Could you check a few things on this drawing? It's one solid part, dimensions in mm from its lowest x, y, z. Give positions to 0.01 mm unless a question says otherwise; leave off trailing zeros. Order: outer loops, then holes, each group sorted by start corner. A loop starts at its lowest first (then second) coordinate and runs counter-clockwise, first axis right, second up. Notation, with made-up numbers: (2.25, -10) -> (9.25, -10) arc R16 cw to (9.25, 13) -> close; hole circle Ø1 at (-37, 19). An arc over 180 degrees is marked (long way). Answer as a JSON object with one key per item and string values.
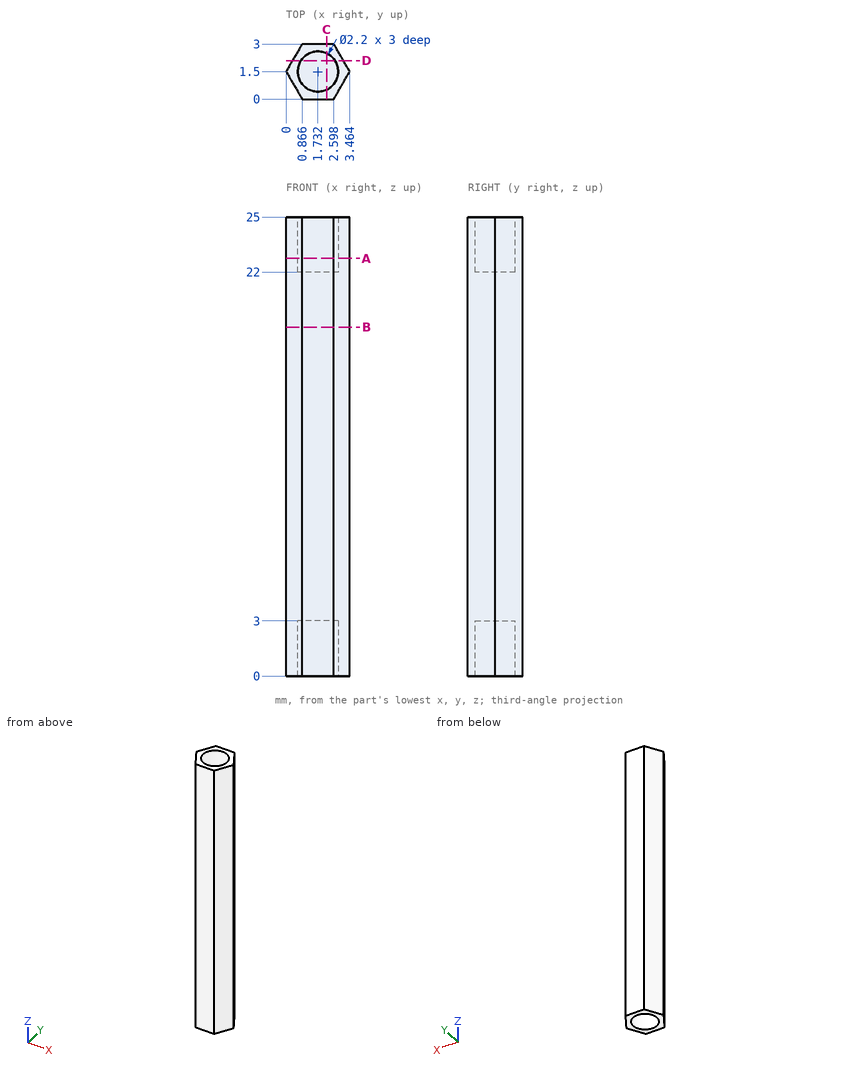
1. If we section it at A-A on z = 22.75: Please give me the cut outline in (x, y).
Worked answers:
{"outline": "(0, 1.5) -> (0.87, 0) -> (2.6, 0) -> (3.46, 1.5) -> (2.6, 3) -> (0.87, 3) -> close; hole circle Ø2.2 at (1.73, 1.5)"}
2. If we section it at B-B on z = 19: Please give me the cut outline in (x, y).
Worked answers:
{"outline": "(0, 1.5) -> (0.87, 0) -> (2.6, 0) -> (3.46, 1.5) -> (2.6, 3) -> (0.87, 3) -> close"}
3. If we section it at C-C on x = 2.2: Please give me the cut outline in (y, z).
Worked answers:
{"outline": "(0, 0) -> (0.5, 0) -> (0.5, 3) -> (2.5, 3) -> (2.5, 0) -> (3, 0) -> (3, 25) -> (2.5, 25) -> (2.5, 22) -> (0.5, 22) -> (0.5, 25) -> (0, 25) -> close"}
4. If we section it at D-D on y = 2.1: Please give me the cut outline in (x, z), then the cut area to 3 significant figures.
Worked answers:
{"outline": "(0.35, 0) -> (0.81, 0) -> (0.81, 3) -> (2.65, 3) -> (2.65, 0) -> (3.12, 0) -> (3.12, 25) -> (2.65, 25) -> (2.65, 22) -> (0.81, 22) -> (0.81, 25) -> (0.35, 25) -> close", "area": "58.2 mm²"}
5. Please list where these lines run through material, in increasing order: L1, parallel to Y at x = 1.8, z = 23.25; L2, parallel to Z at x = 0.7, y = 1.65; L3, parallel to X at y = 0.4, z = 11 (1 decimal).
Worked answers:
{"L1": "0 to 0.4, 2.6 to 3", "L2": "3 to 22", "L3": "0.6 to 2.8"}
